Geometry check sheet. Reference: the model listing, model coordinates, mm. Face numbers are marked on the shaded views. A direction names the side the tool comes from. Coordinates: 2 decimals unless noted, no trailing zeros. Loops run counter-clockwise (first coordinate to the right, second up) from the corner with the lowest first, then second, coordinate; pieces in that order, holes last.
from build123d import *

# Parameters (mm, degrees)
SKETCH_1_W          = 80
SKETCH_1_H          = 150
EXTRUDE_1_DEPTH     = 3
SKETCH_2_W          = 12
SKETCH_2_H          = 22
EXTRUDE_2_DEPTH     = 5
SKETCH_3_R          = 1.9
CUT_EXTRUDE_1_DEPTH = 86.375640554
SKETCH_4_W          = 80
SKETCH_4_H          = 150
SKETCH_4_W_2        = 70.382347564
SKETCH_4_H_2        = 140.764695128
EXTRUDE_3_DEPTH     = 20


with BuildPart() as part:
    # 스케치1 → 보스-돌출1 (new body)
    with BuildSketch(Plane.XY):
        Rectangle(SKETCH_1_W, SKETCH_1_H)
    extrude(amount=EXTRUDE_1_DEPTH)

    # 스케치2 → 보스-돌출2 (add)
    with BuildSketch(Plane.XY):
        Rectangle(SKETCH_2_W, SKETCH_2_H)
    extrude(amount=-EXTRUDE_2_DEPTH)

    # 스케치3 → 컷-돌출1 (cut, through all)
    with BuildSketch(Plane(origin=(0, 0, -5), x_dir=(-1, 0, 0), z_dir=(0, 0, -1))):
        with Locations((0, 5)):
            Circle(SKETCH_3_R)
        with Locations(Location((0, -5, 0), (0, 0, 180))):
            Circle(SKETCH_3_R)
    extrude(amount=-CUT_EXTRUDE_1_DEPTH, mode=Mode.SUBTRACT)

    # 스케치4 → 보스-돌출3 (add)
    with BuildSketch(Plane.XY.offset(3)):
        Rectangle(SKETCH_4_W, SKETCH_4_H)
        Rectangle(SKETCH_4_W_2, SKETCH_4_H_2, mode=Mode.SUBTRACT)
    extrude(amount=EXTRUDE_3_DEPTH)


solid = part.part
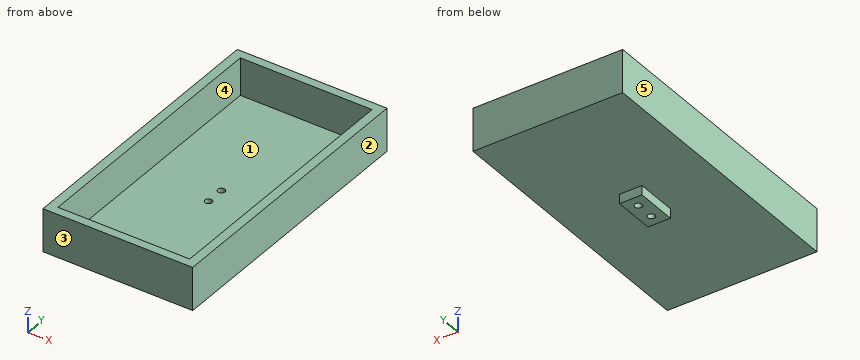
1) Mould release check, pull along X, two halves, no side actions. Record for the marked faces 3, 4 and 5: +X half, -X half, draft (parallel to the pull), parting line (faces both ways), or undercut.
Data:
face 3: draft
face 4: undercut
face 5: -X half
2) Section check C-C on z = 9.5. Record the cut outline in (x, y).
Data:
outline: (-40, -75) - (40, -75) - (40, 75) - (-40, 75) - close; hole (-35.19, -70.38) - (35.19, -70.38) - (35.19, 70.38) - (-35.19, 70.38) - close
3) Material ranges on probe 1 along Y at (x, z) = (0, -1.75); probe 2 along X at (y, z) = (-5, 0.25); probe 3 along X at (y, z) = (-5, -1), recorded low to high.
Data:
probe 1: y = -11 to -6.9, -3.1 to 3.1, 6.9 to 11
probe 2: x = -40 to -1.9, 1.9 to 40
probe 3: x = -6 to -1.9, 1.9 to 6
4) Section check D-D on y = -55.5. Record the cut outline in (x, z).
Data:
outline: (-40, 0) - (40, 0) - (40, 23) - (35.19, 23) - (35.19, 3) - (-35.19, 3) - (-35.19, 23) - (-40, 23) - close
5) Depth check by flat-ended pin: pin 1 (5 mm diameter, centred on x = 0, y = 5, fed in from +Z); pin 2 (2.5 mm diameter, centred on x = -0.5, z = -2.5, fed in from -Y); pin 3 (1.5 mm diameter, centred on y = 4, z = -2, fed in from +X). Enter the tip coordinate at first touch or a pass-through.
Data:
pin 1: stops at z = 3
pin 2: stops at y = -11
pin 3: stops at x = 6
6) Section check B-B on x = 0. Record the cut outline in (y, z), and give its area (3 significant figures).
Data:
outline: (-75, 0) - (-11, 0) - (-11, -5) - (-6.9, -5) - (-6.9, 3) - (-70.38, 3) - (-70.38, 23) - (-75, 23) - close; (-3.1, -5) - (3.1, -5) - (3.1, 3) - (-3.1, 3) - close; (6.9, -5) - (11, -5) - (11, 0) - (75, 0) - (75, 23) - (70.38, 23) - (70.38, 3) - (6.9, 3) - close
area: 684 mm2
7) Section check A-A on y = 5. Record the cut outline in (x, z).
Data:
outline: (-40, 0) - (-6, 0) - (-6, -5) - (-1.9, -5) - (-1.9, 3) - (-35.19, 3) - (-35.19, 23) - (-40, 23) - close; (1.9, -5) - (6, -5) - (6, 0) - (40, 0) - (40, 23) - (35.19, 23) - (35.19, 3) - (1.9, 3) - close
8) Access from +Z, -Z, +X, -X, +Y, -Y to the whole of each face (thin tool, end or side, straight path). Record for the marked faces 1 and 2.
Data:
face 1: +Z
face 2: +Z, -Z, +X, +Y, -Y
